```python
from build123d import *

# Parameters (mm, degrees)
SKETCH1_W                                      = 32
SKETCH1_H                                      = 32
BOSS_EXTRUDE1_DEPTH                            = 7
CSK_FOR_M6_FLAT_HEAD_MACHINE_SCREW1_AT_2_COUNT = 2
CSK_FOR_M6_FLAT_HEAD_MACHINE_SCREW1_AT_2_PITCH = 16


with BuildPart() as part:
    # Sketch1 → Boss-Extrude1 (new body)
    with BuildSketch(Plane(origin=(0, 0, 0), x_dir=(1, 0, 0), z_dir=(0, 1, 0))):
        Rectangle(SKETCH1_W, SKETCH1_H)
    extrude(amount=BOSS_EXTRUDE1_DEPTH)

    # Sketch3 → CSK for M6 Flat Head Machine Screw1 (revolve, cut)
    with BuildSketch(Plane(origin=(-8, 7, 0), x_dir=(0, 0, 1), z_dir=(1, 0, 0))):
        Polygon((0, 0), (0, 7), (3.5, 7), (3.5, 4.849742261), (6.3, 0), align=None)
    csk_for_m6_flat_head_machine_screw1 = revolve(axis=Axis((-8, 13.35, 0), (0, -1, 0)), mode=Mode.SUBTRACT)

    # CSK for M6 Flat Head Machine Screw1 at 2: CSK for M6 Flat Head Machine Screw1 ×2
    with Locations(*[(i * CSK_FOR_M6_FLAT_HEAD_MACHINE_SCREW1_AT_2_PITCH, 0, 0) for i in range(1, CSK_FOR_M6_FLAT_HEAD_MACHINE_SCREW1_AT_2_COUNT)]):
        add(csk_for_m6_flat_head_machine_screw1, mode=Mode.SUBTRACT)


solid = part.part
```
Work out the finished part from the listing and answer in its coordinate system (mm). Round coordinates to 2 decimals unless told otherwise and drop trailing zeros. Write each loop counter-clockwise with the first axis right and the second up, starting at its lowest first coordinate (ties: lowest second). Pieces come first, ordered by that corner, then holes. Notation, with made-up numbers: (-16, 63.25) -> (35, 63.25) arc R25 cw to (35, 99.25) -> close; hole circle Ø7 at (57.25, 48.5). An arc over 180 degrees is marked (long way). Write each question's results on one line, items separated by ' | '.
Q1. Flat-ended cylindrical pins translate along their axes: P1, Ø5.5, axis at x = -8, z = 0, coming from the -Y side; P2, Ø2, axis at x = 6.5, z = 4, coming from the +Y side. Find the tip coordinate at first contact, or state that the pin passes through.
Data:
P1: through | P2: y = 5.22
Q2. Section D-D, the plane y = 2.75 is taken. Write down the section's boundary in (x, z).
Data:
outline: (-16, -16) -> (16, -16) -> (16, 16) -> (-16, 16) -> close; hole circle Ø7.69 at (-8, 0); hole circle Ø7.69 at (8, 0)
Q3. Determine the mould class of faces 1 (the flat face through (16, 3, 0)), 2 (the cylindrical face through (-4.583, 1.09, -0.759)), 3 (the conical face through (6.896, 2.454, 3.505)), 4 (the flat face through (0, 0, 0)) for opening direction X: released by +X, released by -X, zero draft, split by the parting line, or undercut.
Data:
face 1: released by +X | face 2: undercut | face 3: undercut | face 4: zero draft
Q4. Section B-B, the plane z = 0 is taken. Write down the section's boundary in (x, y).
Data:
outline: (-16, 0) -> (-11.5, 0) -> (-11.5, 2.15) -> (-14.3, 7) -> (-16, 7) -> close; (-4.5, 0) -> (4.5, 0) -> (4.5, 2.15) -> (1.7, 7) -> (-1.7, 7) -> (-4.5, 2.15) -> close; (11.5, 0) -> (16, 0) -> (16, 7) -> (14.3, 7) -> (11.5, 2.15) -> close
Q5. Section C-C, the plane y = 0.5 is taken. Write down the section's boundary in (x, z), then the cut area to 3 significant figures.
Data:
outline: (-16, -16) -> (16, -16) -> (16, 16) -> (-16, 16) -> close; hole circle Ø7 at (-8, 0); hole circle Ø7 at (8, 0) | area: 947 mm^2
Q6. Straight lines are drawn through the part: line 1 along X through (y, z) = (0.8, 0); line 2 along X through (y, z) = (5.5, 3.5); line 3 along Z through (x, y) = (-8, 0.6). For each, find the intervals that lie inside material, in ascending order. Write a range as [from, to].
Data:
line 1: [-16, -11.5], [-4.5, 4.5], [11.5, 16] | line 2: [-16, -12.16], [-3.84, 3.84], [12.16, 16] | line 3: [-16, -3.5], [3.5, 16]
Q7. Section A-A, the plane x = 8 is taken. Write down the section's boundary in (y, z), then the cut area to 3 significant figures.
Data:
outline: (0, -16) -> (7, -16) -> (7, -6.3) -> (2.15, -3.5) -> (0, -3.5) -> close; (0, 3.5) -> (2.15, 3.5) -> (7, 6.3) -> (7, 16) -> (0, 16) -> close | area: 161 mm^2
